Could you check a few things on this drawing? It's one solid part, dimensions in mm from its lowest x, y, z. Coordinates: 2 decimals unless noted, no trailing zeros. Loops run counter-clockwise (first coordinate to the right, second up) from the corner with the lowest first, then second, coordinate; pieces in that order, holes last. Notation, with made-up numbers: (25, 32) -> (63, 32) arc R28 cw to (63, 53) -> close; hole circle Ø3 at (-10, -17.75). An arc over 180 degrees is marked (long way). One line per question, with ' | ' between items.
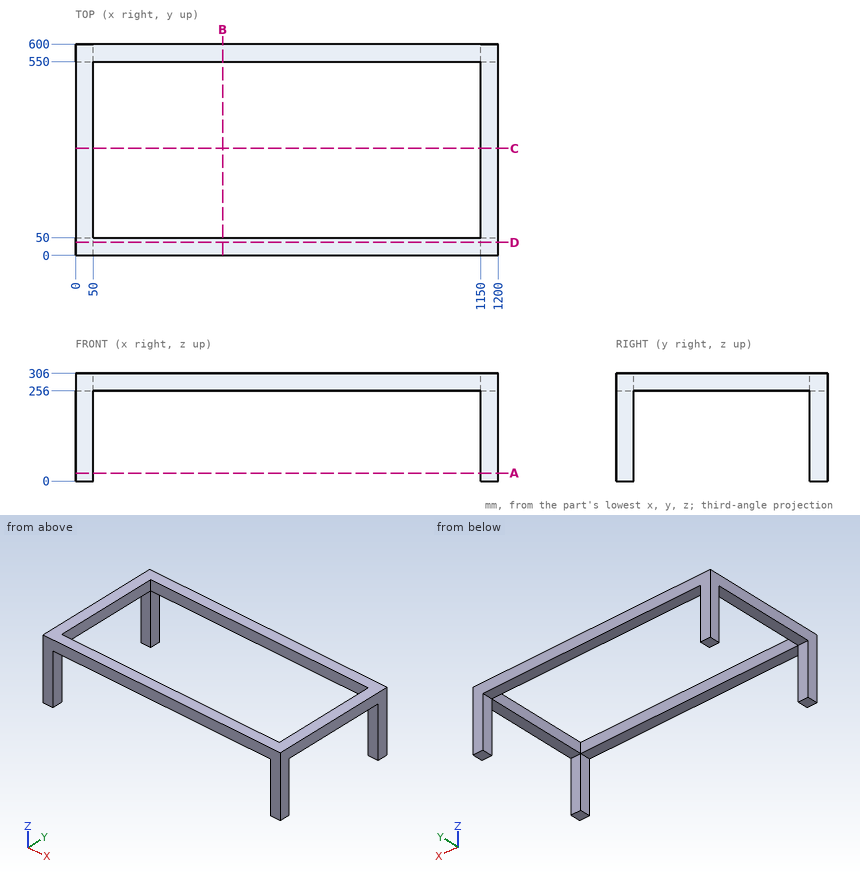
1) If we section it at B-B on x = 417.5: Please give me the cut outline in (y, z), and give its area (3 significant figures).
Data:
outline: (0, 256) -> (50, 256) -> (50, 306) -> (0, 306) -> close; (550, 256) -> (600, 256) -> (600, 306) -> (550, 306) -> close | area: 5,000 mm²
2) I'm going to push a flat-ended pin straight in: pin 1 Ø25 at (x, y) = (718, 580) entering from -Z. Where does the tip first touch, or does it pass through?
Data:
pin 1: z = 256
3) If we section it at A-A on z = 22.5: Please give me the cut outline in (x, y).
Data:
outline: (0, 0) -> (50, 0) -> (50, 50) -> (0, 50) -> close; (0, 550) -> (50, 550) -> (50, 600) -> (0, 600) -> close; (1150, 0) -> (1200, 0) -> (1200, 50) -> (1150, 50) -> close; (1150, 550) -> (1200, 550) -> (1200, 600) -> (1150, 600) -> close
4) If we section it at C-C on y = 304: Please give me the cut outline in (x, z).
Data:
outline: (0, 256) -> (50, 256) -> (50, 306) -> (0, 306) -> close; (1150, 256) -> (1200, 256) -> (1200, 306) -> (1150, 306) -> close
5) I need wall thicknesses on line 1 along X through (y, z) = (524, 283.5); line 2 along Y through (x, z) = (665.5, 273); line 3 along Z through (x, y) = (911.5, 39). Which ranges of each line are inside material? Lowest first, please. Write a range as from..to.
Data:
line 1: 0..50, 1150..1200 | line 2: 0..50, 550..600 | line 3: 256..306
6) If we section it at D-D on y = 37: Please give me the cut outline in (x, z), and give its area (3 significant figures).
Data:
outline: (0, 0) -> (50, 0) -> (50, 256) -> (1150, 256) -> (1150, 0) -> (1200, 0) -> (1200, 306) -> (0, 306) -> close | area: 85,600 mm²
